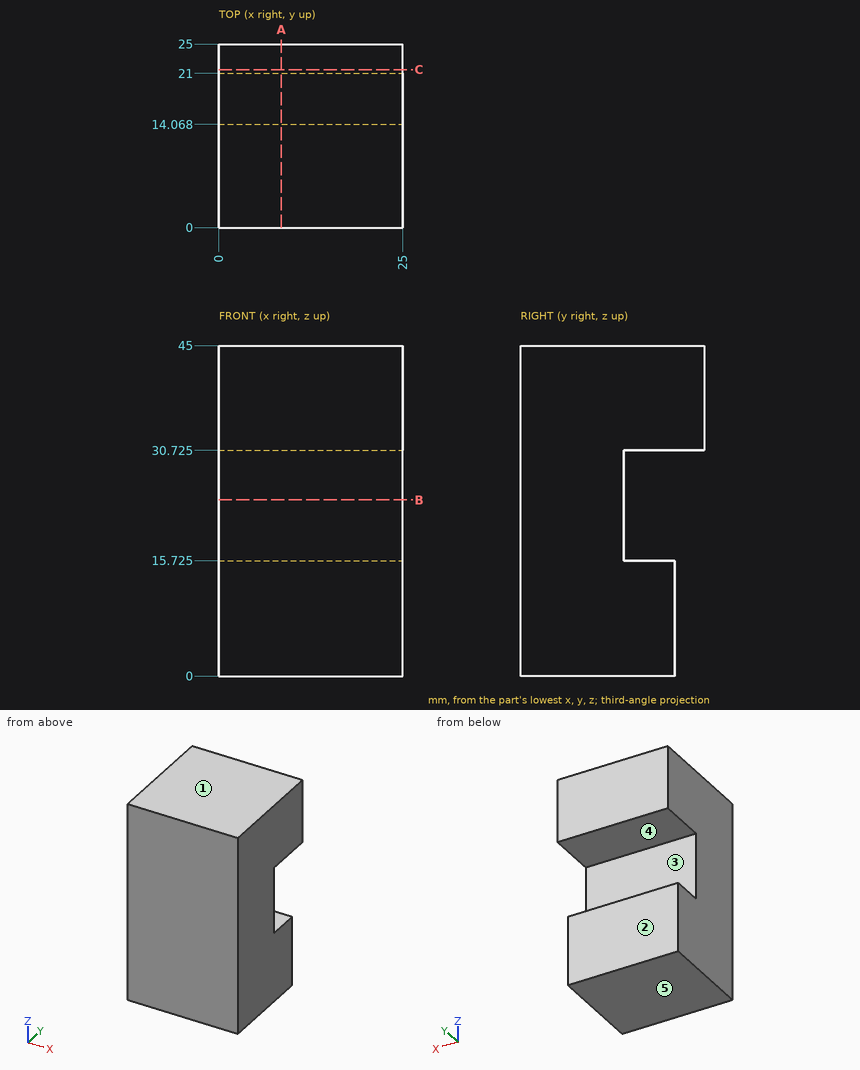
Study the drawing (mm; zero at the part's minimum x, y, z) and answer. A direction names the side the tool comes from. Give positions to 0.01 mm unless a question says otherwise; leave off trailing zeros. Loops run counter-clockwise (first coordinate to the right, second up) from the corner with the lowest first, then second, coordinate; pieces in that order, holes last. Notation, with made-up numbers: M 49,75 L 76,75 A15 ccw 76,104 Z; hole C 26,-27.75 d7. An arc over 180 degrees is marked long. Answer as CSV lines item,"result".
Item 1: The part is cut by section C-C (y = 21.5). Give the vertices of the cut face in (x, z) (3 decimals).
Values follow:
outline,"M 0,30.725 L 25,30.725 L 25,45 L 0,45 Z"
Item 2: The part is cut by section B-B (z = 24). Give the vertices of the cut face in (x, y), and give its area (3 significant figures).
Values follow:
outline,"M 0,0 L 25,0 L 25,14.07 L 0,14.07 Z"
area,"352 mm^2"
Item 3: The part is cut by section A-A (x = 8.5). Give the vertices of the cut face in (y, z) (3 decimals).
Values follow:
outline,"M 0,0 L 21,0 L 21,15.725 L 14.068,15.725 L 14.068,30.725 L 25,30.725 L 25,45 L 0,45 Z"
Item 4: Which of the six approach directions +Z, -Z, +X, -X, +Y, -Y give full straight-line access (tool end or side, diameter ignored) to the marked faces 4 and 5?
Values follow:
face 4,"+X, -X, +Y"
face 5,"-Z, +X, -X, +Y, -Y"
Item 5: The mould has two halves that part along Z. Classify the marked faces 1, 2 and 3: released by +Z, released by -Z, zero draft, split by the parting line, or undercut.
Values follow:
face 1,"released by +Z"
face 2,"zero draft"
face 3,"undercut"
Item 6: Straight lines are drawn through the part: line 1 along Z through (x, y) = (1.25, 20.5) (3 decimals); line 2 along Y through (x, z) = (21.75, 26.5); line 3 along Z through (x, y) = (16.75, 21.25) (3 decimals). For each, find the intervals that lie inside material, in ascending order. Write a range as [from, to].
Values follow:
line 1,"z = [0, 15.725], [30.725, 45]"
line 2,"y = [0, 14.07]"
line 3,"z = [30.725, 45]"
